from build123d import *

# Parameters (mm, degrees)
F0_W     = 38.10014986
F0_H     = 12.7
F1_DEPTH = 50.8
F2_R     = 6.34999
F3_R     = 7.874
F4_DEPTH = 12.701


# Not quite as in the source:
# - a fillet or chamfer is up to 0.001 mm smaller than in the source, because OpenCascade refuses the exact size


with BuildPart() as f1:
    # F0 (on Front) → F1 (new body, symmetric)
    with BuildSketch(Plane.XZ):
        Rectangle(F0_W, F0_H)
    extrude(amount=F1_DEPTH, both=True)

    # F2 (radius 6.35 in the source; OpenCascade refuses exactly that, so slightly less here)
    f2_edges = [f1.edges().sort_by_distance(p)[0] for p in [
        (-19.050075, 0, 6.35),
        (19.050075, 0, 6.35),
        (19.050075, 0, -6.35),
        (-19.050075, 0, -6.35),
    ]]
    fillet(f2_edges, radius=F2_R)

    # F3 (on face) → F4 (cut, through all)
    with BuildSketch(Plane.XY.offset(6.35)):
        with Locations((0, -25.4)):
            Circle(F3_R)
    extrude(amount=-F4_DEPTH, mode=Mode.SUBTRACT)


solid = f1.part
Can you work these out from the model? Positions are in its coordinate system, mm. Coordinates: 2 decimals unless noted, no trailing zeros. Order: outer loops, then holes, each group sorted by start corner. A loop starts at its lowest first (then second) coordinate and runs counter-clockwise, first axis right, second up. Notation, with made-up numbers: M -36,64 L -28,64 A24 cw -28,101 Z; hole C -27,52 d7. An arc over 180 degrees is marked long. Answer as CSV lines item,"result".
(1) If we mould it in two halves opening along X, with no side actions, what happens to faces 1 (the cylindrical face through (3.633, -32.386, 0.089)), 2 (the cylindrical face through (-17.24, -0.71, -4.44)), 3 (the flat face through (0, -1, -6.35))? For each: released by +X, released by -X, zero draft, split by the parting line, or undercut.
Geometry check:
face 1,"undercut"
face 2,"released by -X"
face 3,"zero draft"
(2) I'm going to push flat-ended pins straight in: pin 1 (1 mm diameter, centred on y = -35.5, z = -4.5, fed in from +X); pin 2 (5 mm diameter, centred on y = -27, z = 1, fed in from +X). Where does each tip first touch, or does it pass through?
Geometry check:
pin 1,"x = 17.63"
pin 2,"x = 19.05"
(3) Suppose I cut it at C-C on z = -1. Please give me the cut outline in (x, y), plus the area to 3 significant figures.
Geometry check:
outline,"M -18.97,-50.8 L 18.97,-50.8 L 18.97,50.8 L -18.97,50.8 Z; hole C 0,-25.4 d15.75"
area,"3,660 mm^2"
(4) Suppose I cut it at B-B on x = 0. Please give me the cut outline in (y, z), plus the area to 3 significant figures.
Geometry check:
outline,"M -50.8,-6.35 L -33.27,-6.35 L -33.27,6.35 L -50.8,6.35 Z; M -17.53,-6.35 L 50.8,-6.35 L 50.8,6.35 L -17.53,6.35 Z"
area,"1,090 mm^2"
(5) Please list where these lines run through material, in increasing order: L1, parallel to Y at x = 0, z = 3; L2, parallel to X at y = -4, z = 0.25; L3, parallel to Y at x = -3.5, z = 3.5.
Geometry check:
L1,"-50.8 to -33.27, -17.53 to 50.8"
L2,"-19.05 to 19.05"
L3,"-50.8 to -32.45, -18.35 to 50.8"
